Autodesk Inventor part; units mm, degrees
ref_plane "Work Plane1" through (750, 0, 0) normal (1, 0, 0) x (0, 0, -1)
ref_plane "YZ Plane" through (0, 0, 0) normal (1, 0, 0) x (0, 1, 0)
ref_plane "XZ Plane" through (0, 0, 0) normal (0, 1, 0) x (-1, 0, 0)
sketch "Sketch1" plane through (0, 0, 0) normal (1, 0, 0) x (0, 1, 0)
  circle A0 centre (0, 0) radius 20
  dimension "d0" = 40
extrude "Extrusion1" add sketch "Sketch1" along normal blind 1500
fillet "Fillet1" radius 5 1 edges at (0, -20, 0)
sketch "Sketch2" plane through (0, 0, 0) normal (-1, 0, 0) x (0, 0, 1)
  circle A0 centre (0, 0) radius 7.5
  dimension "d4" = 15
extrude "Extrusion2" add sketch "Sketch2" along normal blind 30
ref_plane "Work Plane1" through (750, 0, 0) normal (1, 0, 0) x (0, 0, -1)
mirror "Mirror1" about plane through (750, 0, 0) normal (1, 0, 0) of "Fillet1", "Extrusion2"
properties part number "CR-1500"
Read the model definition and answer for the solid it produces. Units are mm, in the model's axes. A direction names the side the tool comes from. Coordinates: 2 decimals unless noted, no trailing zeros. Loops run counter-clockwise (first coordinate to the right, second up) from the corner with the lowest first, then second, coordinate; pieces in that order, holes last. Notation, with made-up numbers: (4, 82) -> (27, 82) arc R11 cw to (27, 92) -> close; hole circle Ø2 at (-30, -18.75). An arc over 180 degrees is marked (long way). Return JSON: item names as keys, results as strings.
Item 1: Flat-ended cylindrical pins translate along their axes: P1, Ø1, axis at x = 728.5, z = -11.5, coming from the -Y side; P2, Ø5, axis at x = 805.5, y = -11, coming from the -Z side; P3, Ø5, axis at x = 1167, z = -10, coming from the +Y side. Find the tip coordinate at first contact, or state that the pin passes through.
Answers:
{"P1": "stops at y = -16.7", "P2": "stops at z = -18.1", "P3": "stops at y = 18.54"}
Item 2: Find section A-A (y = 0). Determine the outline of the cut face in (x, z), plus the area to 3 significant figures.
Answers:
{"outline": "(-30, -7.5) -> (0, -7.5) -> (0, -15) arc R5 ccw to (5, -20) -> (1495, -20) arc R5 ccw to (1500, -15) -> (1500, -7.5) -> (1530, -7.5) -> (1530, 7.5) -> (1500, 7.5) -> (1500, 15) arc R5 ccw to (1495, 20) -> (5, 20) arc R5 ccw to (0, 15) -> (0, 7.5) -> (-30, 7.5) -> close", "area": "60,900 mm2"}
Item 3: For faces 1 (the flat face through (1500, -4, 7)), 2 (the flat face through (0, -4, 7)), 3 (the cylindrical face through (739.57, -4.336, 19.524)), determine the directions among +Z, -Z, +X, -X, +Y, -Y from which every point of the face is accessible in a straight line to the end or side of a thin tool.
Answers:
{"face 1": "+X", "face 2": "-X", "face 3": "+X, -X"}
Item 4: Find the intervals of material crossed by probe 1 along X at (y, z) = (-15, -0.5); probe 2 along Y at (x, z) = (414.5, 3); probe 3 along Y at (x, z) = (140, -2), in increasing order.
Answers:
{"probe 1": "x = 0 to 1500", "probe 2": "y = -19.77 to 19.77", "probe 3": "y = -19.9 to 19.9"}
Item 5: Find section C-C (x = 565.5). Determine the outline of the cut face in (y, z), plus the area to 3 significant figures.
Answers:
{"outline": "circle Ø40 at (0, 0)", "area": "1,260 mm2"}
